```python
from build123d import *

# Parameters (mm, degrees)
SKETCH012_R         = 6.75
SKETCH012_R_2       = 5.25
PAD005_DEPTH        = 2
FILLET_R            = 0.75
REVOLUTION002_ANGLE = -50
POLARPATTERN_COUNT  = 5
POLARPATTERN_ANGLE  = 220


with BuildPart() as part:
    # Sketch012 → Pad005 (new body)
    with BuildSketch(Plane.XY):
        Circle(SKETCH012_R)
        Circle(SKETCH012_R_2, mode=Mode.SUBTRACT)
    extrude(amount=PAD005_DEPTH)

    # Fillet
    fillet_edges = [part.edges().sort_by_distance(p)[0] for p in [
        (-6.75, 0, 2),
    ]]
    fillet(fillet_edges, radius=FILLET_R)

    # Sketch013 → Revolution002 (revolve)
    with BuildSketch(Plane(origin=(0, 0, 0), x_dir=(-0.7071067812, -0.7071067812, 0), z_dir=(-0.7071067812, 0.7071067812, 0))):
        with BuildLine():
            Line((7.75, -1.400000012), (7.75, -0.5))
            Line((7.75, -0.5), (6.75, 1.25))
            Line((6.75, 1.25), (6.5642857143, 0))
            Line((6.5642857143, 0), (6.85, -0.5))
            ThreePointArc((6.85, -0.5), (6.2136038927, -2.0363960988), (7.75, -1.400000012))
        make_face()
    revolution002 = revolve(axis=Axis((0, 0, 0), (0, 0, 1)), revolution_arc=REVOLUTION002_ANGLE)

    # PolarPattern: Revolution002 ×5 about axis
    polarpattern_axis = Axis((0, 0, 0), (0, 0, -1))
    for i in range(1, POLARPATTERN_COUNT):
        add(revolution002.rotate(polarpattern_axis, i * POLARPATTERN_ANGLE / (POLARPATTERN_COUNT - 1)))


with BuildPart() as part_1:
    # Body004 placement: moved
    add(part.part.moved(Location((0, 0, 3))))


solid = part_1.part
```
Model file for the job. Use its own axes, mm. A direction names the side the tool comes from. Coordinates: 2 decimals unless noted, no trailing zeros. Write each loop counter-clockwise with the first axis right and the second up, starting at its lowest first coordinate (ties: lowest second). Pieces come first, ordered by that corner, then holes. Notation, with made-up numbers: (-20, 46) - (32, 46) arc R34 cw to (32, 77) - close; hole circle Ø6 at (-34, -21). An arc over 180 degrees is marked (long way). Use a Markdown table: item, result. Add a question column.
Item 1: Drop flat-ended pins along their axis: pin 1 (2 mm diameter, centred on x = 3.5, y = 4, fed in from -Z); pin 2 (1 mm diameter, centred on y = 0, z = 4.5, fed in from +X). Give the stop position or say it passes through.
Item 2: Two-plate mould, pull along X, no slides. Class faces 5 (the face through (-6.375, 4.406, 2.056)), 6 (the face through (7.011, 0.613, 2.105)), 7 (the face through (6.93, 1.22, 2.11)): pulls with the +X half, pulls with the -X half, needs draft (parallel to the pull), parting line crosses it, or undercut.
Item 3: Band-saw the part on A-A, the plane x = 0. Write the cut outline in (y, z).
Item 4: Band-saw the part on B-B, the plane z = 1.9. Give the number of separate pieces and of enclosed holes in the cut face, and give its area (3 significant figures).
Item 5: Band-saw the part on D-D, the plane z = 3.95. Write the cut outline in (x, y) (3 decimals), and give its area (3 significant figures).
Item 6: Band-saw the part on C-C, the plane y = 0. Write the cut outline in (x, z), and give its area (3 significant figures).
Item 7: Drill centre lines: line 1 along Z through (x, y) = (-4, 3.75); line 2 along X through (y, z) = (4.25, 2.85); line 3 along Z through (x, y) = (1.5, 6.25). Where is each one in solid material? Low to high.
Item 8: 3-axis set-ups, long thin cutter, end or side, ignore diameter. For faces 1 (the face through (5.42, 3.84, 2.86)), 2 (the face through (-6.93, 1.22, 2.11)), 3 (the face through (-3.519, 6.095, 2.105)), 4 (the face through (-5, -5, 2)): which of +Z, -Z, +X, -X, +Y, -Y reach the whole face in a straight line?
A:
| question | item | result |
|---|---|---|
| 1 | pin 1 | stops at z = 0.88 |
| 1 | pin 2 | stops at x = 6.89 |
| 2 | face 5 | pulls with the -X half |
| 2 | face 6 | undercut |
| 2 | face 7 | pulls with the +X half |
| 3 | outline | (-6.75, 3) - (-5.25, 3) - (-5.25, 5) - (-6, 5) arc R0.75 ccw to (-6.75, 4.25) - close; (5.25, 3) - (6.56, 3) - (6.85, 2.5) arc R0.9 ccw (long way) to (7.75, 1.6) - (7.75, 2.5) - (6.75, 4.25) arc R0.75 ccw to (6, 5) - (5.25, 5) - close |
| 4 | separate pieces | 5 |
| 4 | enclosed holes | 0 |
| 4 | area | 52.5 mm² |
| 5 | outline | (-6.895, 0.603) arc R6.921 ccw to (-4.894, -4.894) - (-4.773, -4.773) arc R6.75 ccw to (4.773, -4.773) - (4.894, -4.894) arc R6.921 ccw to (6.895, 0.603) - (6.724, 0.588) arc R6.75 ccw to (6.647, 1.172) - (6.816, 1.202) arc R6.921 ccw to (3.461, 5.994) - (3.375, 5.846) arc R6.75 ccw to (2.853, 6.118) - (2.925, 6.273) arc R6.921 ccw to (-2.925, 6.273) - (-2.853, 6.118) arc R6.75 ccw to (-3.375, 5.846) - (-3.461, 5.994) arc R6.921 ccw to (-6.816, 1.202) - (-6.647, 1.172) arc R6.75 ccw to (-6.724, 0.588) - close; hole circle Ø10.5 at (0, 0) |
| 5 | area | 61.7 mm² |
| 6 | outline | (-7.75, 1.6) arc R0.9 ccw (long way) to (-6.85, 2.5) - (-6.56, 3) - (-5.25, 3) - (-5.25, 5) - (-6, 5) arc R0.75 ccw to (-6.75, 4.25) - (-7.75, 2.5) - close; (5.25, 3) - (6.56, 3) - (6.85, 2.5) arc R0.9 ccw (long way) to (7.75, 1.6) - (7.75, 2.5) - (6.75, 4.25) arc R0.75 ccw to (6, 5) - (5.25, 5) - close |
| 6 | area | 13.0 mm² |
| 7 | line 1 | z = 3 to 5 |
| 7 | line 2 | x = -6.24 to -5.11, 5.11 to 6.24 |
| 7 | line 3 | z = 0.81 to 2.39, 3 to 4.87 |
| 8 | face 1 | none |
| 8 | face 2 | -Z, -X |
| 8 | face 3 | -Z |
| 8 | face 4 | -Z, -Y |
